Job drawing, mm, ordinate dimensions from the low corner. One solid piece. A direction names the side the tool comes from. Coordinates: 2 decimals unless noted, no trailing zeros. Write each loop counter-clockwise with the first axis right and the second up, starting at its lowest first coordinate (ties: lowest second). Pieces come first, ordered by that corner, then holes. Notation, with made-up numbers: (13, -19.5) - (68, -19.5) arc R29 cw to (68, 1.5) - close; hole circle Ø7 at (-15, 64). An arc over 180 degrees is marked (long way). Put each result on its own line as item: value. Start each with the question number.
1. Drop flat-ended pins along their axis: P1, Ø4, axis at x = 27.5, z = 33.5, coming from the +Y side; P2, Ø4, axis at x = 6.5, z = 22.5, coming from the +Y side; P3, Ø5, axis at x = 15.5, y = 30.5, coming from the +Z side. Give the stop position or say it passes through.
2. Saw through at A-A, the plane y = 23.5. Write the cut outline in (x, z).
3. Which spindle directions (+Z, -Z, +X, -X, +Y, -Y) get a long thin tool onto all of the face, cutting with end or side? Do the marked faces 5, 6 and 7. Say none if no direction does.
4. Pull direction Y, two halves, no side cores. Call the marked faces 1, 2, 3 and 4: released by +Y, released by -Y, zero draft, split by the parting line, or undercut.
5. Drill centre lines: L1, parallel to X at y = 16.5, z = 13.5; L2, parallel to Z at x = 17, y = 3.5; L3, parallel to X at y = 5, z = 34. Where is each one in solid material? Low to high. Write a range as from..to.
6. Saw through at C-C, the plane z = 4. Write the cut outline in (x, y).
7. Saw through at B-B, the plane z = 22. Write the cut outline in (x, y), plus the area to 4 significant figures.
8. Saw through at D-D, the plane y = 37.5. Write the cut outline in (x, z).
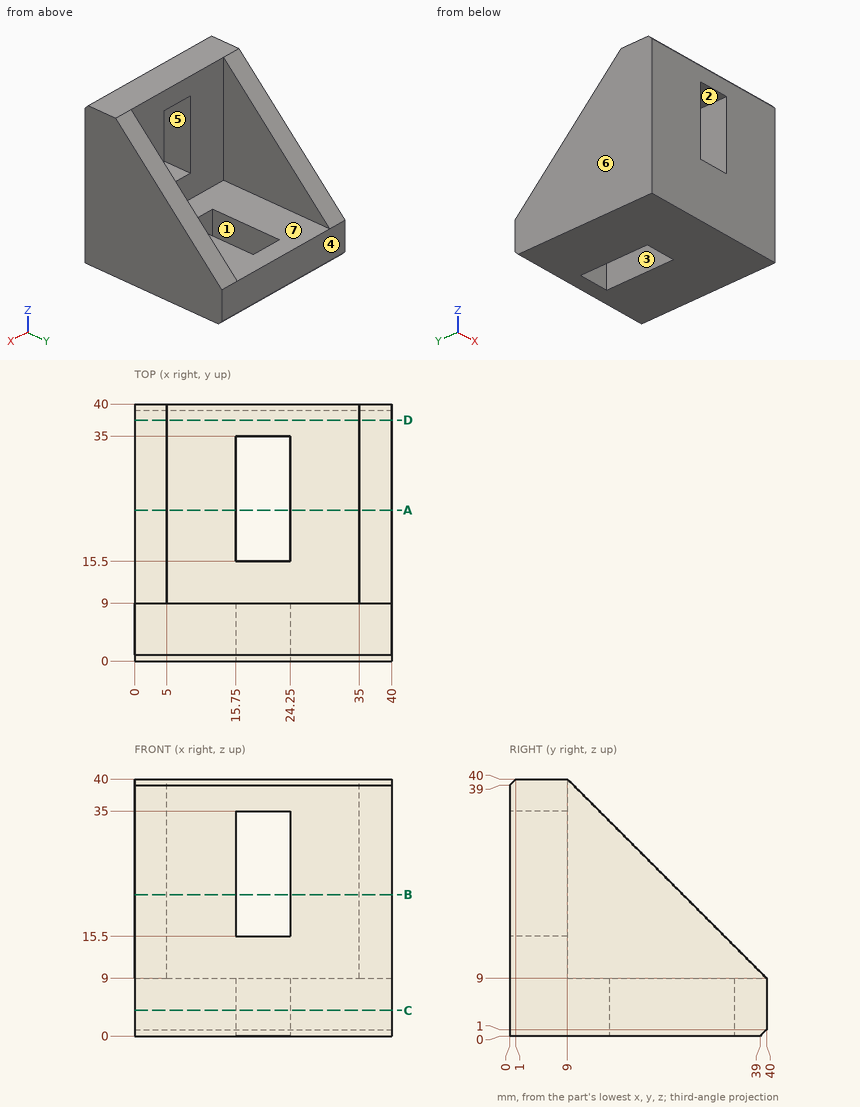
Final values:
1. P1: stops at y = 9
1. P2: stops at y = 27.82
1. P3: stops at z = 9
2. outline: (0, 0) - (15.75, 0) - (15.75, 9) - (5, 9) - (5, 25.5) - (0, 25.5) - close; (24.25, 0) - (40, 0) - (40, 25.5) - (35, 25.5) - (35, 9) - (24.25, 9) - close
3. face 5: +Y, -Y
3. face 6: +Z, -Z, -X, +Y, -Y
3. face 7: +Z, +Y
4. face 1: undercut
4. face 2: zero draft
4. face 3: undercut
4. face 4: released by +Y
5. L1: x = 0..5, 35..40
5. L2: z = 0..15.5, 35..40
5. L3: x = 0..15.75, 24.25..40
6. outline: (0, 0) - (40, 0) - (40, 40) - (0, 40) - close; hole (15.75, 15.5) - (24.25, 15.5) - (24.25, 35) - (15.75, 35) - close
7. outline: (0, 0) - (15.75, 0) - (15.75, 9) - (5, 9) - (5, 27) - (0, 27) - close; (24.25, 0) - (40, 0) - (40, 27) - (35, 27) - (35, 9) - (24.25, 9) - close
7. area: 463.5 mm²
8. outline: (0, 0) - (40, 0) - (40, 11.5) - (35, 11.5) - (35, 9) - (5, 9) - (5, 11.5) - (0, 11.5) - close
